Part model, mm, in its own coordinate system. Face numbers are marked on the shaded views. Give positions to 0.01 mm unless a question says otherwise; leave off trailing zeros. Order: outer loops, then holes, each group sorted by start corner. A loop starts at its lowest first (then second) coordinate and runs counter-clockwise, first axis right, second up. Notation, with made-up numbers: (44, -7) - (86, -7) arc R16 ccw to (86, 19) - close; hole circle Ø6 at (-15, 67). An arc over 180 degrees is marked (long way). One line per item, written item: value.
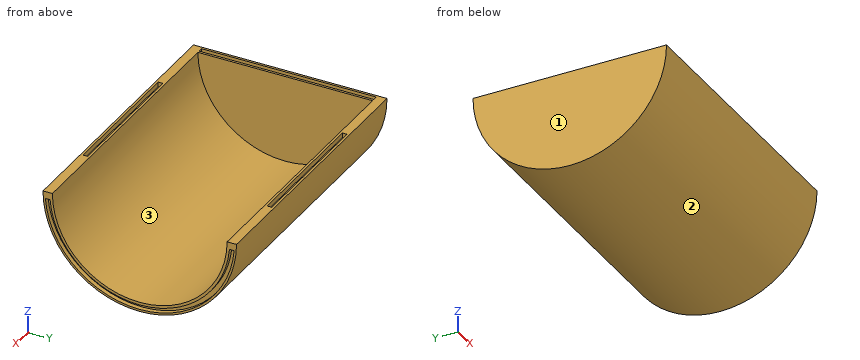
```python
from build123d import *

# Parameters (mm, degrees)
REVOLVE1_ANGLE     = 180
SKETCH4_W          = 2.54
SKETCH4_H          = 94.488
SKETCH4_W_2        = 76.2
SKETCH4_H_2        = 2.54
CUT_EXTRUDE1_DEPTH = 2.54
CUT_EXTRUDE2_DEPTH = 2.54


with BuildPart() as part:
    # Sketch1 → Revolve1 (revolve)
    with BuildSketch(Plane.XY):
        Polygon((0, 0), (0, 52.324), (152.4, 52.324), (152.4, 47.244), (5.08, 47.244), (5.08, 0), align=None)
    revolve(axis=Axis((5.08, 0, 0), (-1, 0, 0)), revolution_arc=REVOLVE1_ANGLE)

    # Sketch4 → Cut-Extrude1 (cut)
    with BuildSketch(Plane.XY):
        with Locations((2.54, 0)):
            Rectangle(SKETCH4_W, SKETCH4_H)
        with Locations((76.2, 49.784)):
            Rectangle(SKETCH4_W_2, SKETCH4_H_2)
        with Locations((76.2, -49.784)):
            Rectangle(SKETCH4_W_2, SKETCH4_H_2)
    extrude(amount=-CUT_EXTRUDE1_DEPTH, mode=Mode.SUBTRACT)

    # Sketch5 → Cut-Extrude2 (cut)
    with BuildSketch(Plane(origin=(152.4, 0, 0), x_dir=(0, 0, -1), z_dir=(1, 0, 0))):
        with BuildLine():
            Line((3.81, 51.054), (3.81, 48.514))
            ThreePointArc((3.81, 48.514), (48.663377359, 0), (3.81, -48.514))
            Line((3.81, -48.514), (3.81, -51.054))
            ThreePointArc((3.81, -51.054), (51.195966794, 0), (3.81, 51.054))
        make_face()
    extrude(amount=-CUT_EXTRUDE2_DEPTH, mode=Mode.SUBTRACT)


solid = part.part
```
1) Cut at B-B, the plane x = 76. Give the cut face in (y, z).
Outcome:
outline: (-52.32, 0) arc R52.32 ccw to (52.32, 0) - (51.05, 0) - (51.05, -2.54) - (48.51, -2.54) - (48.51, 0) - (47.24, 0) arc R47.24 cw to (-47.24, 0) - (-48.51, 0) - (-48.51, -2.54) - (-51.05, -2.54) - (-51.05, 0) - close
2) Cut at C-C, the plane z = -29. Give the cut face in (x, y), then the cut area to 3 significant figures.
Outcome:
outline: (0, -43.55) - (152.4, -43.55) - (152.4, -42.19) - (149.86, -42.19) - (149.86, -39.08) - (152.4, -39.08) - (152.4, -37.3) - (5.08, -37.3) - (5.08, 37.3) - (152.4, 37.3) - (152.4, 39.08) - (149.86, 39.08) - (149.86, 42.19) - (152.4, 42.19) - (152.4, 43.55) - (0, 43.55) - close
area: 2,270 mm^2
3) Pin check, flat tips, straight feed: pin 1 (12 mm diameter, centred on x = 91.5, y = 3, fed in from -Z); pin 2 (23.5 mm diameter, centred on y = -0.5, z = -27, fed in from +X); pin 3 (0.8 mm diameter, centred on x = 92, y = 50.5, fed in from +Z). Stop position of each tip, or through.
Outcome:
pin 1: stops at z = -52.32
pin 2: stops at x = 5.08
pin 3: stops at z = -2.54
4) Cut at A-A, the plane y = 0. Give the cut face in (x, z), then the cut area to 3 significant figures.
Outcome:
outline: (0, -52.32) - (152.4, -52.32) - (152.4, -51.2) - (149.86, -51.2) - (149.86, -48.66) - (152.4, -48.66) - (152.4, -47.24) - (5.08, -47.24) - (5.08, 0) - (3.81, 0) - (3.81, -2.54) - (1.27, -2.54) - (1.27, 0) - (0, 0) - close
area: 1,000 mm^2
5) Cut at D-D, the plane y = 44. Give the cut face in (x, z).
Outcome:
outline: (0, -28.32) - (152.4, -28.32) - (152.4, -26.17) - (149.86, -26.17) - (149.86, -20.79) - (152.4, -20.79) - (152.4, -17.2) - (5.08, -17.2) - (5.08, 0) - (3.81, 0) - (3.81, -2.54) - (1.27, -2.54) - (1.27, 0) - (0, 0) - close
6) Drill centre lines: line 1 along X through (y, z) = (-27, -25); line 2 along Y through (x, z) = (94, -23); line 3 along Y through (x, z) = (10, -30). Where is each one in solid material? Low to high. Write a range as from..to.
Outcome:
line 1: x = 0..5.08
line 2: y = -47..-41.27, 41.27..47
line 3: y = -42.87..-36.5, 36.5..42.87
7) Mould opens along Y. For the marked faces 1, 2 and 3 say: released by +Y, released by -Y, zero draft, split by the parting line, or undercut.
Outcome:
face 1: zero draft
face 2: split by the parting line
face 3: undercut
